```python
from build123d import *

# Parameters (mm, degrees)
F1_DEPTH = 63.5
F2_DEPTH = 25.4
F3_DEPTH = 7.9375
F0_W     = 25.2205249548
F0_H     = 19.0500000358
F5_R     = 6.35


with BuildPart() as f1:
    # F0 (on Front) → F1 (new body, symmetric)
    with BuildSketch(Plane.XZ):
        Polygon((-41.275, -9.525), (41.275, -9.525), (41.275, 9.525), (22.2249999642, 9.525), (-41.275, 9.525), align=None)
    extrude(amount=F1_DEPTH, both=True)

    # F0 (on Front) → F2 (join, symmetric)
    with BuildSketch(Plane.XZ):
        with BuildLine():
            Line((22.2249999642, 9.525), (41.275, 9.525))
            Line((41.275, 9.525), (41.275, 27.0002))
            ThreePointArc((41.275, 27.0002), (45.9246798487, 38.2255201513), (57.15, 42.8752))
            Line((57.15, 42.8752), (60.325, 42.8752))
            Line((60.325, 42.8752), (60.325, 61.9252000358))
            Line((60.325, 61.9252000358), (57.15, 61.9252000358))
            ThreePointArc((57.15, 61.9252000358), (32.4542956418, 51.6959043582), (22.2249999642, 27.0002))
            Line((22.2249999642, 27.0002), (22.2249999642, 9.525))
        make_face()
    extrude(amount=F2_DEPTH, both=True)

    # F0 (on Front) → F3 (join, symmetric)
    with BuildSketch(Plane.XZ):
        with BuildLine():
            add(Edge.make_bspline(
                [(-41.275, 9.525), (-40.8977142173, 34.432549157), (0, 61.9252000358), (57.15, 61.9252000358)],
                knots=[0, 0, 0, 0, 111.5045361803, 111.5045361803, 111.5045361803, 111.5045361803], degree=3))
            Line((-41.275, 9.525), (22.2249999642, 9.525))
            Line((22.2249999642, 9.525), (22.2249999642, 27.0002))
            ThreePointArc((22.2249999642, 27.0002), (32.4542956418, 51.6959043582), (57.15, 61.9252000358))
        make_face()
    extrude(amount=F3_DEPTH, both=True)

    # F0 (on Front) → F4 (revolve)
    with BuildSketch(Plane.XZ):
        with Locations((72.9352624774, 52.4002000179)):
            Rectangle(F0_W, F0_H)
    revolve(axis=Axis((60.325, 0, 52.3875), (0, 0, 1)))

    # F5
    f5_edges = [f1.edges().sort_by_distance(p)[0] for p in [
        (41.275, -63.5, 0),
        (-41.275, -63.5, 0),
        (41.275, 63.5, 0),
        (-41.275, 63.5, 0),
    ]]
    fillet(f5_edges, radius=F5_R)


solid = f1.part
```
Geometry check sheet. Reference: the model listing, model coordinates, mm. A direction names the side the tool comes from. Coordinates: 2 decimals unless noted, no trailing zeros. Order: outer loops, then holes, each group sorted by start corner. A loop starts at its lowest first (then second) coordinate and runs counter-clockwise, first axis right, second up.
Q1. Depth check by flat-ended pin: pin 1 Ø5 at (x, z) = (5, 20) entering from +Y; pin 2 Ø8.5 at (y, z) = (14.5, 19.5) entering from -X (3 decimals); pin 3 Ø19 at (x, z) = (44.5, 27.5) entering from +Y. Enter the tip coordinate at first touch or a pass-through.
Reply:
pin 1: stops at y = 7.94
pin 2: stops at x = 22.225
pin 3: stops at y = 25.4
Q2. Sectioned sample at B-B on x = 68. Record the cut outline in (y, z).
Reply:
outline: (-24.02, 42.88) - (24.02, 42.88) - (24.02, 61.93) - (-24.02, 61.93) - close
Q3. Thickness scan on probe 1 along Y at (x, z) = (41, 38.5); probe 2 along Z at (x, y) = (-17.5, -47.5) (3 decimals); probe 3 along Z at (x, y) = (76, 1). Record the ranges inside material, lowest first.
Reply:
probe 1: y = -25.4 to 25.4
probe 2: z = -9.525 to 9.525
probe 3: z = 42.88 to 61.93
Q4. Tool access check on faces 1 (the face through (28.763, -16.791, 47.346)), 2 (the face through (1, 35, 9.525)), 3 (the face through (35.11, 0.51, 60.83)). Record the directions out of +Z, -Z, +X, -X, +Y, -Y that give a thin tool (end or side, any length) a straight path to the whole face; none if there is none.
Reply:
face 1: +Z, -X, -Y
face 2: +Z, -X, +Y
face 3: +Z, -X
Q5. Sectioned sample at A-A on y = 29.5. Record the cut outline in (x, z) (3 decimals).
Reply:
outline: (-41.275, -9.525) - (41.275, -9.525) - (41.275, 9.525) - (-41.275, 9.525) - close
